Here's the drawing with two shaded views (mm, measured from the low corner). I have some questions. Give positions to 0.01 mm unless a question says otherwise; leave off trailing zeros. Loops run counter-clockwise (first coordinate to the right, second up) from the corner with the lowest first, then second, coordinate; pieces in that order, holes last. Notation, with made-up numbers: M 25,33 L 30,33 A20 cw 30,43 Z; hole C 85,11 d9. An arc over 180 degrees is marked long. Use a Markdown table: item, result. Add a question column.
1) If I drill on line 1 along Y through (x, z) = (4.75, 5); line 2 along Y through (x, z) = (5, 4.25), over which ranges is the centre line in solid material (lowest first)? Write a range as [from, to].
2) Suppose I cut it at C-C on x = 5.5. List the corners of the cut face in (y, z) for me, and give its area (3 significant figures).
3) Suppose I cut it at D-D on z = 5.5. List the corners of the cut face in (x, y) for me, and give its area (3 significant figures).
4) Suppose I cut it at B-B on z = 15. List the corners of the cut face in (x, y) for me, and give its area (4 significant figures).
5) Suppose I cut it at A-A on y = 2. List the corners of the cut face in (x, z) for me.
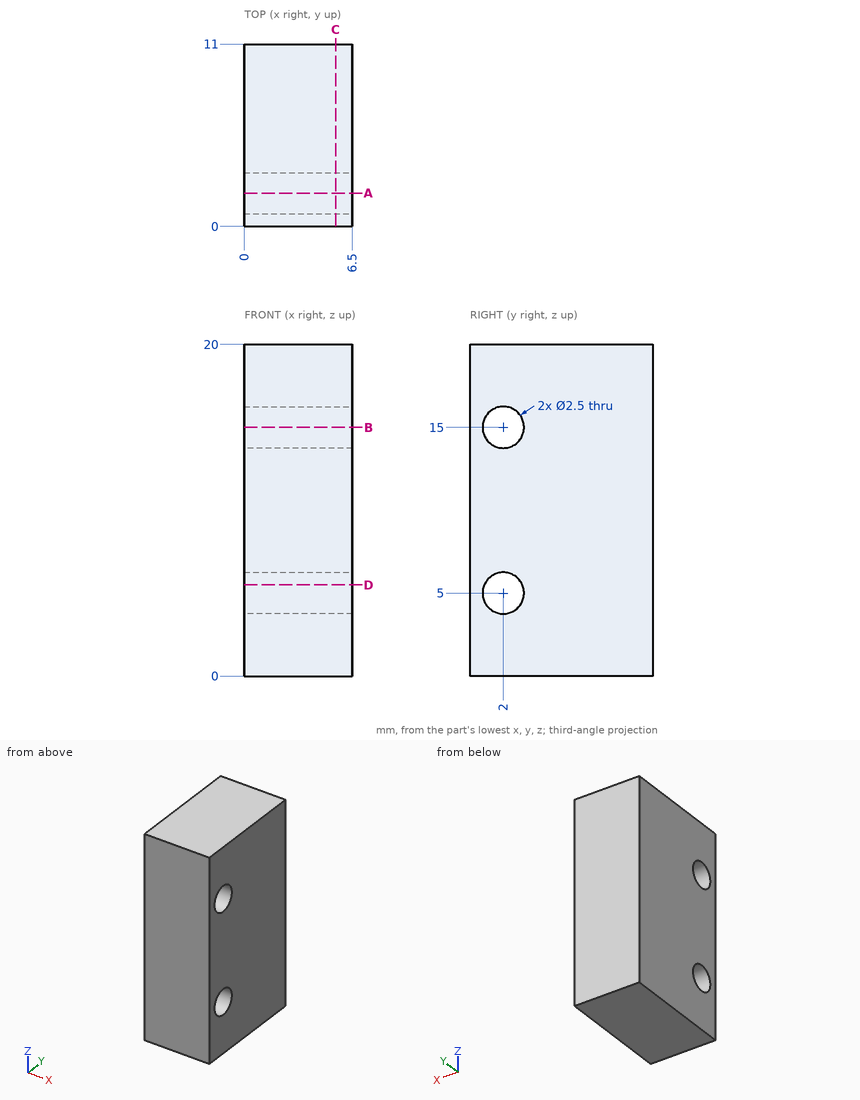
Answer block:
| question | item | result |
|---|---|---|
| 1 | line 1 | y = [0, 0.75], [3.25, 11] |
| 1 | line 2 | y = [0, 1], [3, 11] |
| 2 | outline | M 0,0 L 11,0 L 11,20 L 0,20 Z; hole C 2,5 d2.5; hole C 2,15 d2.5 |
| 2 | area | 210 mm^2 |
| 3 | outline | M 0,0 L 6.5,0 L 6.5,0.85 L 0,0.85 Z; M 0,3.15 L 6.5,3.15 L 6.5,11 L 0,11 Z |
| 3 | area | 56.6 mm^2 |
| 4 | outline | M 0,0 L 6.5,0 L 6.5,0.75 L 0,0.75 Z; M 0,3.25 L 6.5,3.25 L 6.5,11 L 0,11 Z |
| 4 | area | 55.25 mm^2 |
| 5 | outline | M 0,0 L 6.5,0 L 6.5,3.75 L 0,3.75 Z; M 0,6.25 L 6.5,6.25 L 6.5,13.75 L 0,13.75 Z; M 0,16.25 L 6.5,16.25 L 6.5,20 L 0,20 Z |
